Part model, mm, in its own coordinate system. Face numbers are marked on the shaded views. Give positions to 0.01 mm unless a question says otherwise; leave off trailing zeros. Order: outer loops, then holes, each group sorted by start corner. A loop starts at its lowest first (then second) coordinate and runs counter-clockwise, first axis right, second up. Notation, with made-up numbers: M 0,13.25 L 35,13.25 A21 ccw 35,31.25 Z; hole C 6,-14.5 d6. An arc over 180 degrees is marked long. One line per question, with ' | ' between items.
```python
from build123d import *

# Parameters (mm, degrees)
F0_R     = 10
F0_R_2   = 3.175
F1_DEPTH = 15
F2_R     = 5
F3_DEPTH = 10
F4_R     = 0.508


with BuildPart() as f1:
    # F0 (on Top) → F1 (new body, symmetric)
    with BuildSketch(Plane.XY):
        Circle(F0_R)
        Circle(F0_R_2, mode=Mode.SUBTRACT)
    extrude(amount=F1_DEPTH, both=True)

    # F2 (on face) → F3 (cut)
    with BuildSketch(Plane.XY.offset(15)):
        Circle(F2_R)
    extrude(amount=-F3_DEPTH, mode=Mode.SUBTRACT)

    # F4
    f4_edges = [f1.edges().sort_by_distance(p)[0] for p in [
        (-10, 0, 15),
        (-10, 0, -15),
    ]]
    fillet(f4_edges, radius=F4_R)


solid = f1.part
```
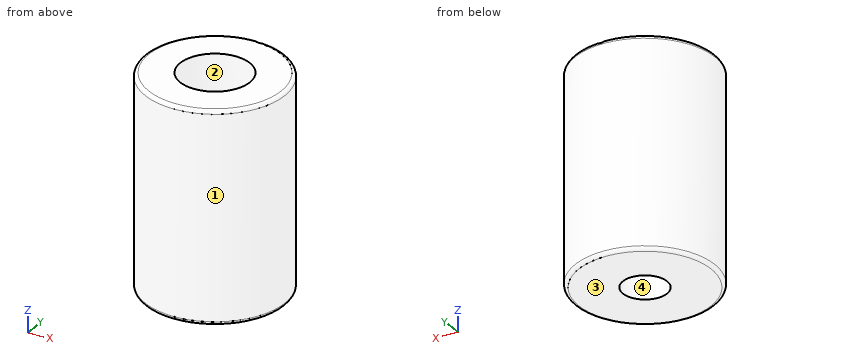
1. Mould opens along Y. For the marked faces 1, 2, 3 and 4 say: released by +Y, released by -Y, zero draft, split by the parting line, or undercut.
Worked out:
face 1: split by the parting line | face 2: undercut | face 3: zero draft | face 4: undercut
2. Slice it at A-A on x = 0. Give the cut face in (y, z) (3 decimals), then the cut area to 3 significant figures.
Worked out:
outline: M -10,-14.492 A0.508 ccw -9.492,-15 L -3.175,-15 L -3.175,5 L -5,5 L -5,15 L -9.492,15 A0.508 ccw -10,14.492 Z; M 3.175,-15 L 9.492,-15 A0.508 ccw 10,-14.492 L 10,14.492 A0.508 ccw 9.492,15 L 5,15 L 5,5 L 3.175,5 Z | area: 373 mm2
3. Drop flat-ended pins along their axis: pin 1 (4 mm diameter, centred on x = 3, z = 11.5, fed in from +Y); pin 2 (3 mm diameter, centred on y = -8, z = 8, fed in from -X); pin 3 (9 mm diameter, centred on x = 0, y = 0, fed in from +Z). Give the stop position or say it passes through.
Worked out:
pin 1: stops at y = 9.95 | pin 2: stops at x = -7.6 | pin 3: stops at z = 5
4. Slice it at D-D on z = 7.5. Give the cut face in (x, y), then the cut area to 3 significant figures.
Worked out:
outline: C 0,0 d20; hole C 0,0 d10 | area: 236 mm2
5. Probe L1, parallel to Y at x = 0, z = 9; L2, parallel to Y at x = 0, z = -4.5 (3 decimals); L3, parallel to X at y = -2.75, z = 11.75. List the from-to ranges inside material, lowest first. Write a range as from..to.
Worked out:
L1: y = -10..-5, 5..10 | L2: y = -10..-3.175, 3.175..10 | L3: x = -9.61..-4.18, 4.18..9.61
6. Slice it at C-C on z = 0. Give the cut face in (x, y) (3 decimals).
Worked out:
outline: C 0,0 d20; hole C 0,0 d6.35
